Verification items for the finished model (mm, model axes). Round coordinates to 2 decimals unless told otherwise and drop trailing zeros. Order: outer loops, then holes, each group sorted by start corner. A loop starts at its lowest first (then second) coordinate and runs counter-clockwise, first axis right, second up. Notation, with made-up numbers: (-13, 19) -> (18, 19) arc R17 ccw to (18, 35) -> close; hole circle Ø1 at (19, 17.25). An arc over 180 degrees is marked (long way). Write item = value, one per line. Start each with the question number.
from build123d import *

# Parameters (mm, degrees)
SKETCH2_W           = 254
SKETCH2_H           = 203.2
BOSS_EXTRUDE1_DEPTH = 5.08
SKETCH4_R           = 19.939
CUT_EXTRUDE2_DEPTH  = 326.318376979
SKETCH3_R           = 8.89
CUT_EXTRUDE3_DEPTH  = 326.318376979


with BuildPart() as part:
    # Sketch2 → Boss-Extrude1 (new body)
    with BuildSketch(Plane.XY):
        with Locations((127, 101.6)):
            Rectangle(SKETCH2_W, SKETCH2_H)
    extrude(amount=BOSS_EXTRUDE1_DEPTH)

    # Sketch4 → Cut-Extrude2 (cut, through all)
    with BuildSketch(Plane.XY.offset(5.08)):
        with Locations((127, 101.6)):
            Circle(SKETCH4_R)
    extrude(amount=-CUT_EXTRUDE2_DEPTH, mode=Mode.SUBTRACT)

    # Sketch3 → Cut-Extrude3 (cut, through all)
    with BuildSketch(Plane.XY.offset(5.08)):
        with Locations((12.7, 190.5)):
            Circle(SKETCH3_R)
        with Locations((241.3, 190.5)):
            Circle(SKETCH3_R)
        with Locations((127, 12.7)):
            Circle(SKETCH3_R)
    extrude(amount=-CUT_EXTRUDE3_DEPTH, mode=Mode.SUBTRACT)


solid = part.part
(1) Cross-section at B-B (y = 190.5). Enter the section's corners in (x, z), and give its area (3 significant figures).
(2) Cross-section at A-A (x = 241.3). Enter the section's corners in (y, z).
(3) Scan lines: line 1 along Y through (x, z) = (127, 1.3); line 2 along Y through (x, z) = (241.3, 1.35); line 3 along Y through (x, z) = (240, 1.85). Record each from-to range of solid material in increasing order. Write a range as from..to.
(4) Cross-section at D-D (y = 12.7). Enter the section's corners in (x, z).
(5) Draft check along Y on faces 1 (the flat face through (125, 203.2, 3)), 2 (the flat face through (125, 0, 3)), 3 (the flat face through (125, 80, 5.08)), 4 (the cylindrical face through (118.12, 13.09, 2.58)). Enter one of: +Y half, -Y half, draft (parallel to the pull), parting line (faces both ways), or undercut.
(6) Cross-section at C-C (x = 127). Enter the section's corners in (y, z), and give its area (3 significant figures).
Outcome:
q1.outline = (0, 0) -> (3.81, 0) -> (3.81, 5.08) -> (0, 5.08) -> close; (21.59, 0) -> (232.41, 0) -> (232.41, 5.08) -> (21.59, 5.08) -> close; (250.19, 0) -> (254, 0) -> (254, 5.08) -> (250.19, 5.08) -> close
q1.area = 1,110 mm^2
q2.outline = (0, 0) -> (181.61, 0) -> (181.61, 5.08) -> (0, 5.08) -> close; (199.39, 0) -> (203.2, 0) -> (203.2, 5.08) -> (199.39, 5.08) -> close
q3.line_1 = 0..3.81, 21.59..81.66, 121.54..203.2
q3.line_2 = 0..181.61, 199.39..203.2
q3.line_3 = 0..181.71, 199.29..203.2
q4.outline = (0, 0) -> (118.11, 0) -> (118.11, 5.08) -> (0, 5.08) -> close; (135.89, 0) -> (254, 0) -> (254, 5.08) -> (135.89, 5.08) -> close
q5.face_1 = +Y half
q5.face_2 = -Y half
q5.face_3 = draft
q5.face_4 = undercut
q6.outline = (0, 0) -> (3.81, 0) -> (3.81, 5.08) -> (0, 5.08) -> close; (21.59, 0) -> (81.66, 0) -> (81.66, 5.08) -> (21.59, 5.08) -> close; (121.54, 0) -> (203.2, 0) -> (203.2, 5.08) -> (121.54, 5.08) -> close
q6.area = 739 mm^2
